```python
from build123d import *

# Parameters (mm, degrees)
SKETCH_1_R          = 1
EXTRUDE_1_DEPTH     = 32.5
SKETCH_2_R          = 3
EXTRUDE_2_DEPTH     = 3.5
SKETCH_3_R          = 10
EXTRUDE_3_DEPTH     = 3
SKETCH_4_R          = 5
EXTRUDE_4_DEPTH     = 1
SKETCH_5_R          = 1
CUT_EXTRUDE_1_DEPTH = 3
SKETCH_6_W          = 52.078633919
SKETCH_6_H          = 39.097037898
CUT_EXTRUDE_2_DEPTH = 32.5


with BuildPart() as part:
    # ｽｹｯﾁ1 → ﾎﾞｽ - 押し出し1 (new body)
    with BuildSketch(Plane.XY):
        with BuildLine():
            Line((-17.482907979, 4.845565749), (13.517092021, 4.845565749))
            ThreePointArc((13.517092021, 4.845565749), (20.100097265, 3.428570993), (25.517092021, -0.571429007))
            Line((25.517092021, -0.571429007), (25.517092021, -21.737439495))
            ThreePointArc((25.517092021, -21.737439495), (20.100097265, -25.737439495), (13.517092021, -27.154434251))
            Line((13.517092021, -27.154434251), (-17.482907979, -27.154434251))
            Line((-17.482907979, -27.154434251), (-17.482907979, 4.845565749))
        make_face()
        with Locations((-14.482907979, -24.654434251)):
            Circle(SKETCH_1_R, mode=Mode.SUBTRACT)
        with Locations((12.517092021, -24.654434251)):
            Circle(SKETCH_1_R, mode=Mode.SUBTRACT)
        with Locations((12.517092021, 2.345565749)):
            Circle(SKETCH_1_R, mode=Mode.SUBTRACT)
        with Locations((-14.482907979, 2.345565749)):
            Circle(SKETCH_1_R, mode=Mode.SUBTRACT)
    extrude(amount=EXTRUDE_1_DEPTH)

    # ｽｹｯﾁ2 → ﾎﾞｽ - 押し出し2 (add)
    with BuildSketch(Plane.XY.offset(32.5)):
        with Locations((13.517092021, -11.154434251)):
            Circle(SKETCH_2_R)
    extrude(amount=EXTRUDE_2_DEPTH)

    # ｽｹｯﾁ3 → ﾎﾞｽ - 押し出し3 (add)
    with BuildSketch(Plane.XY.offset(36)):
        with Locations((13.517092021, -11.154434251)):
            Circle(SKETCH_3_R)
    extrude(amount=-EXTRUDE_3_DEPTH)

    # ｽｹｯﾁ4 → ﾎﾞｽ - 押し出し4 (add)
    with BuildSketch(Plane.XY.offset(36)):
        with Locations((13.517092021, -11.154434251)):
            Circle(SKETCH_4_R)
    extrude(amount=EXTRUDE_4_DEPTH)

    # ｽｹｯﾁ5 → ｶｯﾄ - 押し出し1 (cut)
    with BuildSketch(Plane.XY.offset(36)):
        with Locations((20.517092021, -11.154434251)):
            Circle(SKETCH_5_R)
        with Locations((18.466839489, -16.104181719)):
            Circle(SKETCH_5_R)
        with Locations((13.517092021, -18.154434251)):
            Circle(SKETCH_5_R)
        with Locations((8.567344553, -16.104181719)):
            Circle(SKETCH_5_R)
        with Locations((6.517092021, -11.154434251)):
            Circle(SKETCH_5_R)
        with Locations((8.567344553, -6.204686782)):
            Circle(SKETCH_5_R)
        with Locations((13.517092021, -4.154434251)):
            Circle(SKETCH_5_R)
        with Locations((18.466839489, -6.204686782)):
            Circle(SKETCH_5_R)
    extrude(amount=-CUT_EXTRUDE_1_DEPTH, mode=Mode.SUBTRACT)

    # ｽｹｯﾁ6 → ｶｯﾄ - 押し出し2 (cut)
    with BuildSketch(Plane(origin=(0, 0, 0), x_dir=(-1, 0, 0), z_dir=(0, 0, -1))):
        with Locations((-8.556408981, -7.605915302)):
            Rectangle(SKETCH_6_W, SKETCH_6_H)
    extrude(amount=-CUT_EXTRUDE_2_DEPTH, mode=Mode.SUBTRACT)


solid = part.part
```
For this review, take the finished solid that the model builds, in its own axes (mm). A direction names the side the tool comes from. Round coordinates to 2 decimals unless told otherwise and drop trailing zeros. Write each loop counter-clockwise with the first axis right and the second up, starting at its lowest first coordinate (ties: lowest second). Pieces come first, ordered by that corner, then holes. Notation, with made-up numbers: (-13.75, -28) - (9.25, -28) arc R12 cw to (9.25, -16) - close; hole circle Ø3 at (-38.5, -17). An arc over 180 degrees is marked (long way). Answer as CSV lines item,"result". Start each with the question number.
(1) Mouldability with a two-part tool opening along Y and no side actions: class faces 4 (the flat face through (14, -11, 32.5)), 5 (the cylindrical face through (16.379, -10.253, 32.746)), 6 (the cylindrical face through (13.387, -17.163, 34.521)) as +Y half, -Y half, draft (parallel to the pull), parting line (faces both ways), or undercut.
(2) For line 1 (X direction, y = -6.75, z = 34.4); line 2 (Y direction, x = 9, z = 33.75); line 3 (Z direction, x = 6.75, y = -4), list the stretches that pass through material, from the lowest coordinate up.
(3) Add section D-D, the plane z = 33.45. State how many separate pieces and enclosed holes the cut face has, plus the area to 3 significant figures.
(4) Add section A-A, the plane x = 8.75. State the section outline as (y, z) points, plus the area to 3 significant figures.
(5) Add section C-C, the plane y = -9.25. State the section outline as (x, z) points.
(6) Machinability: for faces 1 (the flat face through (11.15, -6.57, 36)), 2 (the cylindrical face through (7.05, -10.31, 34.52)), 3 (the flat face through (16, -9, 33)), which of the approach directions +Z, -Z, +X, -X, +Y, -Y give a long, thin tool a straight path to every point of the face, cutting with its end or side? Answer none if there is none.
(7) Add section B-B, the plane x = 6.5. State the section outline as (y, z) points.
(8) For pin 1 (3 mm diameter, centred on x = 6.52, y = -11.15, fed in from +Z); pin 2 (3 mm diameter, centred on x = 8.57, y = -6.2, fed in from -Z); pin 3 (1.5 mm diameter, centred on y = -19, z = 33, fed in from -X), all flat-tipped, find the tip position at first contact; note any pin that passes through.
From the geometry:
1,face 4,"draft"
1,face 5,"parting line"
1,face 6,"undercut"
2,line 1,"x = 4.54 to 7.73, 9.41 to 17.63, 19.31 to 22.49"
2,line 2,"y = -20.08 to -17.01, -15.2 to -7.11, -5.3 to -2.23"
2,line 3,"z = 33 to 36"
3,separate pieces,"1"
3,enclosed holes,"8"
3,area,"289 mm²"
4,outline,"(-19.95, 33) - (-17.09, 33) - (-17.09, 36) - (-19.95, 36) - close; (-15.12, 33) - (-7.19, 33) - (-7.19, 36) - (-9.65, 36) - (-9.65, 37) - (-12.66, 37) - (-12.66, 36) - (-15.12, 36) - close; (-5.22, 33) - (-2.36, 33) - (-2.36, 36) - (-5.22, 36) - close"
4,area,"44.0 mm²"
5,outline,"(3.7, 33) - (11.2, 33) - (11.2, 32.5) - (15.84, 32.5) - (15.84, 33) - (23.33, 33) - (23.33, 36) - (18.14, 36) - (18.14, 37) - (8.89, 37) - (8.89, 36) - (3.7, 36) - close"
6,face 1,"+Z"
6,face 2,"+Z, -Z"
6,face 3,"-Z"
7,outline,"(-18.28, 33) - (-12.15, 33) - (-12.15, 36) - (-18.28, 36) - close; (-10.15, 33) - (-4.03, 33) - (-4.03, 36) - (-10.15, 36) - close"
8,pin 1,"stops at z = 36"
8,pin 2,"stops at z = 33"
8,pin 3,"stops at x = 6.47"
